Check sheet for the modelled part. Datum: model origin and axes. Units: mm. A direction names the side the tool comes from. Coordinates: 2 decimals unless noted, no trailing zeros. Loops run counter-clockwise (first coordinate to the right, second up) from the corner with the lowest first, then second, coordinate; pieces in that order, holes last. Notation, with made-up numbers: (-32.5, 21.5) -> (-10.5, 21.5) arc R8 ccw to (-10.5, 35.5) -> close; hole circle Ø5 at (51.5, -34.5). An arc over 180 degrees is marked (long way). Use CSV: the item, a comma, the result in double quotes.
```python
from build123d import *

# Parameters (mm, degrees)
PAD001_DEPTH    = 10
SKETCH005_W     = 9.25
SKETCH005_H     = 5
PAD002_DEPTH    = 30
SKETCH006_R     = 1.5
POCKET001_DEPTH = 11


with BuildPart() as part:
    # Sketch002 → Pad001 (new body)
    with BuildSketch(Plane.XY):
        with BuildLine():
            Line((-39.757408, -23.461055), (-19.235308, -23.461055))
            ThreePointArc((-19.235308, -23.461055), (-16.591471, -22.365942), (-15.496358, -19.722105))
            Line((-15.496358, -19.722105), (-15.496358, -18.461055))
            Line((-15.496358, -18.461055), (-6.246358, -18.461055))
            Line((-6.246358, -18.461055), (-6.246358, -27.461055))
            Line((-6.246358, -27.461055), (-112.246358, -27.461055))
            Line((-112.246358, -27.461055), (-112.246358, -43.461055))
            Line((-112.246358, -43.461055), (-6.246358, -43.461055))
            Line((-6.246358, -43.461055), (-6.246358, -47.461055))
            Line((-6.246358, -47.461055), (-116.246358, -47.461055))
            Line((-116.246358, -47.461055), (-116.246358, -23.461055))
            Line((-116.246358, -23.461055), (-56.485308, -23.461055))
            ThreePointArc((-56.485308, -23.461055), (-53.841471, -22.365942), (-52.746358, -19.722105))
            Line((-52.746358, -19.722105), (-52.746358, -18.461055))
            Line((-52.746358, -18.461055), (-43.496358, -18.461055))
            Line((-43.496358, -18.461055), (-43.496358, -19.722105))
            ThreePointArc((-43.496358, -19.722105), (-42.401245, -22.365942), (-39.757408, -23.461055))
        make_face()
    extrude(amount=PAD001_DEPTH)

    # Sketch005 → Pad002 (new body)
    with BuildSketch(Plane.XY.offset(10)):
        with Locations((-10.871358, -20.961055)):
            Rectangle(SKETCH005_W, SKETCH005_H)
        with Locations((-48.121358, -20.961055)):
            Rectangle(SKETCH005_W, SKETCH005_H)
    extrude(amount=PAD002_DEPTH)

    # Sketch006 → Pocket001 (cut)
    with BuildSketch(Plane.XZ.offset(23.461055)):
        with Locations((-46.746358, 28.9)):
            Circle(SKETCH006_R)
        with Locations((-11.746358, 28.9)):
            Circle(SKETCH006_R)
    extrude(amount=-POCKET001_DEPTH, mode=Mode.SUBTRACT)


solid = part.part
```
1) Access from +Z, -Z, +X, -X, +Y, -Y to the whole of each face (thin tool, end or side, straight path). Record for faces 1 (the flat face through (-87, -23.461, 5)), 2 (the flat face through (-48, -23.461, 25)), 3 (the flat face through (-48, -18.461, 20)).
Answer below:
face 1,"+Z, -Z, -X, +Y"
face 2,"+Z, +X, -X, -Y"
face 3,"+Z, -Z, +X, -X, +Y"
2) Draft check along X on faces 4 (the cylindrical face through (-42.43, -22.337, 4.93)), 5 (the cylindrical face through (-53.871, -22.395, 4.93)), 6 (the flat face through (-112.246, -35, 5)). Enter one of: released by +X, released by -X, zero draft, split by the parting line, or undercut.
Answer below:
face 4,"undercut"
face 5,"released by -X"
face 6,"released by +X"
3) Cross-section at C-C on z = 22. Record the boundary of the cut face in (x, y), and give its area (3 significant figures).
Answer below:
outline,"(-52.75, -23.46) -> (-43.5, -23.46) -> (-43.5, -18.46) -> (-52.75, -18.46) -> close; (-15.5, -23.46) -> (-6.25, -23.46) -> (-6.25, -18.46) -> (-15.5, -18.46) -> close"
area,"92.5 mm²"
4) Cross-section at A-A on z = 28.9. Record the boundary of the cut face in (x, y), and give its area (3 significant figures).
Answer below:
outline,"(-52.75, -23.46) -> (-48.25, -23.46) -> (-48.25, -18.46) -> (-52.75, -18.46) -> close; (-45.25, -23.46) -> (-43.5, -23.46) -> (-43.5, -18.46) -> (-45.25, -18.46) -> close; (-15.5, -23.46) -> (-13.25, -23.46) -> (-13.25, -18.46) -> (-15.5, -18.46) -> close; (-10.25, -23.46) -> (-6.25, -23.46) -> (-6.25, -18.46) -> (-10.25, -18.46) -> close"
area,"62.5 mm²"
5) Go/stop test with flat-tipped pins: pin 1 Ø5.5 at (y, z) = (-21.5, 23.5) entering from -X; pin 2 Ø7.5 at (x, z) = (-49.5, 28) entering from -Y; pin 3 Ø3 at (x, z) = (-86, 4.5) entering from +Y. Record where each tip stops, or that it passes through.
Answer below:
pin 1,"stops at x = -52.75"
pin 2,"stops at y = -23.46"
pin 3,"stops at y = -23.46"
6) Thickness scan on line 1 along Z through (x, y) = (-51, -26.5); line 2 along Y through (x, z) = (-13, 19); line 3 along X through (y, z) = (-39.75, 6). Record the ranges inside material, lowest first. Write a range as from..to.
Answer below:
line 1,"z = 0..10"
line 2,"y = -23.46..-18.46"
line 3,"x = -116.25..-112.25"
7) Cross-section at B-B on x = -69.5. Record the boundary of the cut face in (y, z), and give its area (3 significant figures).
Answer below:
outline,"(-47.46, 0) -> (-43.46, 0) -> (-43.46, 10) -> (-47.46, 10) -> close; (-27.46, 0) -> (-23.46, 0) -> (-23.46, 10) -> (-27.46, 10) -> close"
area,"80.0 mm²"
8) Cross-section at D-D on z = 7. Record the boundary of the cut face in (x, y).
Answer below:
outline,"(-116.25, -47.46) -> (-6.25, -47.46) -> (-6.25, -43.46) -> (-112.25, -43.46) -> (-112.25, -27.46) -> (-6.25, -27.46) -> (-6.25, -18.46) -> (-15.5, -18.46) -> (-15.5, -19.72) arc R3.74 cw to (-19.24, -23.46) -> (-39.76, -23.46) arc R3.74 cw to (-43.5, -19.72) -> (-43.5, -18.46) -> (-52.75, -18.46) -> (-52.75, -19.72) arc R3.74 cw to (-56.49, -23.46) -> (-116.25, -23.46) -> close"
